Part model, mm, in its own coordinate system. A direction names the side the tool comes from. Give positions to 0.01 mm unless a question says otherwise; leave off trailing zeros. Order: outer loops, then holes, each group sorted by start corner. A loop starts at its lowest first (then second) coordinate and runs counter-clockwise, first axis right, second up. Notation, with made-up numbers: (6, -28) -> (56, -28) arc R28 cw to (56, 0) -> close; hole circle Ø1 at (59.5, -22.75). An arc over 180 degrees is marked (long way). Write item = value, one per line. Start each with the question number.
(1) Saw through at C-C, the plane x = -20. List the corners of the cut face in (y, z).
(2) Probe line 1 along Y through (x, z) = (0, 1.3); line 2 along Y through (x, z) = (-20, 12.25); line 3 along Y through (x, z) = (27, 11.5). List the from-to ranges inside material, lowest first. Write a range as from..to.
(3) Two-plate mould, pull along Y, no slides. Class faces 1 (the cylindrical face through (18.71, 21.18, 2.46)), 2 (the flat face through (0, 27, 0)), 3 (the flat face through (-22.48, 34.405, 0.986)), 4 (the flat face through (0, 28, 10)): pulls with the +Y half, pulls with the -Y half, needs draft (parallel to the pull), parting line crosses it, or undercut.
(4) Saw through at A-A, the plane z = 1. List the corners of the cut face in (x, y), then the cut area to 3 significant figures.
(5) Saw through at D-D, the plane z = 8.25. List the corners of the cut face in (x, y), then the cut area to 3 significant figures.
(6) Saw through at B-B, the plane y = 0. List the corners of the cut face in (x, z).
(7) Which spindle directions (+Z, -Z, +X, -X, +Y, -Y) get a long thin tool onto all of the face, cutting with end or side? Do faces 5 (the flat face through (-17.54, 34.44, 0.99)), 6 (the flat face through (0, 33, 15)). Say none if no direction does.
(8) Flat gauge pins, fed straight in: pin 1 (3 mm diameter, centred on x = 20, y = -20, fed in from -Z); pin 2 (4 mm diameter, centred on y = -3, z = 3.5, fed in from +X); pin 3 (2 mm diameter, centred on x = 16, z = 13, fed in from -Y); pin 4 (1.6 mm diameter, centred on x = 19.5, z = 0.5, fed in from -Y). Where does each tip first touch, or does it go through?
from build123d import *

# Parameters (mm, degrees)
ESQUISSE1_W             = 55
ESQUISSE1_H             = 56
ESQUISSE1_R             = 1.75
ESQUISSE1_R_2           = 24
BOSS_EXTRU_1_DEPTH      = 5
CONG_1_R                = 15
ESQUISSE2_W             = 70
ESQUISSE2_H             = 10
BOSS_EXTRU_2_DEPTH      = 10
ESQUISSE3_R             = 1.75
ENL_V_MAT_EXTRU_1_DEPTH = 26
ENL_V_MAT_EXTRU_2_DEPTH = 2
CONG_2_R                = 10


with BuildPart() as part:
    # Esquisse1 → Boss.-Extru.1 (new body)
    # profile 1 of 2: a face of its own
    with BuildSketch(Plane.XY):
        Rectangle(ESQUISSE1_W, ESQUISSE1_H)
        with Locations((-20, -20)):
            Circle(ESQUISSE1_R, mode=Mode.SUBTRACT)
        with Locations((20, -20)):
            Circle(ESQUISSE1_R, mode=Mode.SUBTRACT)
        with Locations((20, 20)):
            Circle(ESQUISSE1_R, mode=Mode.SUBTRACT)
        with Locations((-20, 20)):
            Circle(ESQUISSE1_R, mode=Mode.SUBTRACT)
        Circle(ESQUISSE1_R_2, mode=Mode.SUBTRACT)
    # profile 2 of 2: a face of its own
    with BuildSketch(Plane.XY):
        Polygon((-35, 28), (-27.5, 28), (27.5, 28), (35, 28), (35, 38), (-35, 38), align=None)
    extrude(amount=BOSS_EXTRU_1_DEPTH)

    # Congé1
    cong_1_edges = [part.edges().sort_by_distance(p)[0] for p in [
        (27.5, -28, 2.5),
        (-27.5, -28, 2.5),
    ]]
    fillet(cong_1_edges, radius=CONG_1_R)

    # Esquisse2 → Boss.-Extru.2 (add)
    with BuildSketch(Plane.XY.offset(5)):
        with Locations((0, 33)):
            Rectangle(ESQUISSE2_W, ESQUISSE2_H)
    extrude(amount=BOSS_EXTRU_2_DEPTH)

    # Esquisse3 → Enlèv. mat.-Extru.1 (cut)
    with BuildSketch(Plane.XY.offset(15)):
        with Locations((-20, 33)):
            Circle(ESQUISSE3_R)
        with Locations((20, 33)):
            Circle(ESQUISSE3_R)
    extrude(amount=-ENL_V_MAT_EXTRU_1_DEPTH, mode=Mode.SUBTRACT)

    # Esquisse4 → Enlèv. mat.-Extru.2 (cut)
    with BuildSketch(Plane(origin=(0, 0, 0), x_dir=(-1, 0, 0), z_dir=(0, 0, -1))):
        Polygon((-16.709103466, 33), (-18.354551733, 35.85), (-21.645448267, 35.85), (-23.290896534, 33), (-21.645448267, 30.15), (-18.354551733, 30.15), align=None)
        Polygon((16.709103466, 33), (18.354551733, 30.15), (21.645448267, 30.15), (23.290896534, 33), (21.645448267, 35.85), (18.354551733, 35.85), align=None)
    extrude(amount=-ENL_V_MAT_EXTRU_2_DEPTH, mode=Mode.SUBTRACT)

    # Congé2
    # the kernel refuses this fillet: 10 mm, written as the material it adds along each edge
    with BuildSketch(Plane(origin=(-27.5, 28, 0), x_dir=(0, -1, 0), z_dir=(0, 0, 1))) as cong_2_piece_1:
        with BuildLine():
            CenterArc((9.682458366, -10), CONG_2_R, 90, 75.522487814)
            Line((0, -7.5), (-0.193649167, -7.45))
            ThreePointArc((-0.193649167, -7.45), (-0.2, -3.75), (-0.2, 0))
            Line((-0.2, 0), (0, 0.2))
            Line((0, 0.2), (9.682458366, 0.2))
            Line((9.682458366, 0.2), (9.682458366, 0))
        make_face()
    extrude(amount=5)
    with BuildSketch(Plane(origin=(27.5, 28, 0), x_dir=(1, 0, 0), z_dir=(0, 0, 1))) as cong_2_piece_2:
        with BuildLine():
            CenterArc((10, -9.682458366), CONG_2_R, 104.477512186, 75.522487814)
            Line((0, -9.682458366), (-0.2, -9.682458366))
            Line((-0.2, -9.682458366), (-0.2, 0))
            Line((-0.2, 0), (0, 0.2))
            ThreePointArc((0, 0.2), (3.75, 0.2), (7.45, 0.193649167))
            Line((7.45, 0.193649167), (7.5, 0))
        make_face()
    extrude(amount=5)


solid = part.part
Results list:
q1.outline = (-25.99, 0) -> (-21.75, 0) -> (-21.75, 5) -> (-25.99, 5) -> close; (-18.25, 0) -> (-13.27, 0) -> (-13.27, 5) -> (-18.25, 5) -> close; (13.27, 0) -> (18.25, 0) -> (18.25, 5) -> (13.27, 5) -> close; (21.75, 0) -> (30.15, 0) -> (30.15, 2) -> (31.25, 2) -> (31.25, 15) -> (28, 15) -> (28, 5) -> (21.75, 5) -> close; (34.75, 2) -> (35.85, 2) -> (35.85, 0) -> (38, 0) -> (38, 15) -> (34.75, 15) -> close
q2.line_1 = -28..-24, 24..38
q2.line_2 = 28..31.25, 34.75..38
q2.line_3 = 28..38
q3.face_1 = undercut
q3.face_2 = needs draft
q3.face_3 = undercut
q3.face_4 = pulls with the -Y half
q4.outline = (-35, 28) arc R10 cw to (-27.5, 18.32) -> (-27.5, -13) arc R15 ccw to (-12.5, -28) -> (12.5, -28) arc R15 ccw to (27.5, -13) -> (27.5, 18.32) arc R10 cw to (35, 28) -> (35, 38) -> (-35, 38) -> close; hole circle Ø48 at (0, 0); hole (-23.29, 33) -> (-21.65, 30.15) -> (-18.35, 30.15) -> (-16.71, 33) -> (-18.35, 35.85) -> (-21.65, 35.85) -> close; hole circle Ø3.5 at (-20, -20); hole circle Ø3.5 at (-20, 20); hole (16.71, 33) -> (18.35, 30.15) -> (21.65, 30.15) -> (23.29, 33) -> (21.65, 35.85) -> (18.35, 35.85) -> close; hole circle Ø3.5 at (20, -20); hole circle Ø3.5 at (20, 20)
q4.area = 1,820 mm^2
q5.outline = (-35, 28) -> (35, 28) -> (35, 38) -> (-35, 38) -> close; hole circle Ø3.5 at (-20, 33); hole circle Ø3.5 at (20, 33)
q5.area = 681 mm^2
q6.outline = (-27.5, 0) -> (-24, 0) -> (-24, 5) -> (-27.5, 5) -> close; (24, 0) -> (27.5, 0) -> (27.5, 5) -> (24, 5) -> close
q7.face_5 = -Z
q7.face_6 = +Z, +X, -X, +Y, -Y
q8.pin_1 = through
q8.pin_2 = 27.5
q8.pin_3 = 28
q8.pin_4 = -26.66
